Input: part model. Units: mm. Frame: model coordinates. Face numbers are marked on the shaded views. A direction names the side the tool comes from. Give positions to 0.01 mm unless a question says otherwise; leave off trailing zeros. Loops run counter-clockwise (first coordinate to the right, second up) from the corner with the lowest first, then second, coordinate; pieces in that order, holes last. Notation, with made-up numbers: (25, 50) -> (82, 50) arc R23 ccw to (82, 79) -> close; hole circle Ø8 at (6, 77.25). An arc over 180 degrees is marked (long way). One line per question, with ' | ' between items.
from build123d import *

# Parameters (mm, degrees)
F0_W     = 44
F0_H     = 44
F1_DEPTH = 25
F0_W_2   = 264
F0_H_2   = 264
F4_DEPTH = 50
F5_DEPTH = 44
F6_DEPTH = 22
F7_SIZE  = 21.99999


# Not quite as in the source:
# - a fillet or chamfer is up to 0.001 mm smaller than in the source, because OpenCascade refuses the exact size


with BuildPart() as f1:
    # F0 (on Top) → F1 (new body)
    with BuildSketch(Plane.XY):
        with Locations((-88, 88)):
            Rectangle(F0_W, F0_H)
    extrude(amount=F1_DEPTH)


with BuildPart() as f1b:
    # F0 (on Top) → F1, piece 2 (new body)
    with BuildSketch(Plane.XY):
        with Locations((0, 88)):
            Rectangle(F0_W, F0_H)
    extrude(amount=F1_DEPTH)


with BuildPart() as f1c:
    # F0 (on Top) → F1, piece 3 (new body)
    with BuildSketch(Plane.XY):
        Rectangle(F0_W, F0_H)
    extrude(amount=F1_DEPTH)


with BuildPart() as f1d:
    # F0 (on Top) → F1, piece 4 (new body)
    with BuildSketch(Plane.XY):
        with Locations((-88, 0)):
            Rectangle(F0_W, F0_H)
    extrude(amount=F1_DEPTH)


with BuildPart() as f2_1:
    # F2: instance of F1d
    add(f1d.part.mirror(Plane.YZ))


with BuildPart() as f2_2:
    # F2: instance of F1
    add(f1.part.mirror(Plane.YZ))


with BuildPart() as f3_1:
    # F3: instance of F1
    add(f1.part.mirror(Plane.XZ))


with BuildPart() as f3_2:
    # F3: instance of F1b
    add(f1b.part.mirror(Plane.XZ))


with BuildPart() as f3_3:
    # F3: instance of F2_2
    add(f2_2.part.mirror(Plane.XZ))


with BuildPart() as f1_1:
    add(f1.part)

    add(f1b.part)  # F4 merges F1b

    add(f1c.part)  # F4 merges F1c

    add(f1d.part)  # F4 merges F1d

    add(f2_1.part)  # F4 merges F2_1

    add(f2_2.part)  # F4 merges F2_2

    add(f3_1.part)  # F4 merges F3_1

    add(f3_2.part)  # F4 merges F3_2

    add(f3_3.part)  # F4 merges F3_3
    # F0 (on Top) → F4 (join)
    with BuildSketch(Plane.XY):
        Rectangle(F0_W_2, F0_H_2)
        with Locations((-88, 0)):
            Rectangle(F0_W, F0_H, mode=Mode.SUBTRACT)
        with Locations((-88, 88)):
            Rectangle(F0_W, F0_H, mode=Mode.SUBTRACT)
        Rectangle(F0_W, F0_H, mode=Mode.SUBTRACT)
        with Locations((0, 88)):
            Rectangle(F0_W, F0_H, mode=Mode.SUBTRACT)
        with Locations((-88, 0)):
            Rectangle(F0_W, F0_H)
        Rectangle(F0_W, F0_H)
        with Locations((-88, 88)):
            Rectangle(F0_W, F0_H)
        with Locations((0, 88)):
            Rectangle(F0_W, F0_H)
    extrude(amount=-F4_DEPTH)

    # F5 (add): faces of the model
    f5_faces = [f1_1.faces().sort_by_distance(p)[0] for p in [
        (-88, -66, 12.5),
        (-88, 22, 12.5),
        (0, 22, 12.5),
        (0, -66, 12.5),
        (88, -66, 12.5),
        (88, 22, 12.5),
    ]]
    extrude(f5_faces, amount=F5_DEPTH)

    # F6 (add, symmetric): faces of the model
    f6_faces = [f1_1.faces().sort_by_distance(p)[0] for p in [
        (-88, -110, 12.5),
        (0, -110, 12.5),
        (88, -110, 12.5),
        (-88, 110, 12.5),
        (0, 110, 12.5),
        (88, 110, 12.5),
    ]]
    extrude(f6_faces, amount=F6_DEPTH, both=True, dir=(0, -1, 0))

    # F7 (size 22 in the source; OpenCascade refuses exactly that, so slightly less here)
    f7_edges = [f1_1.edges().sort_by_distance(p)[0] for p in [
        (-110, 0, 25),
        (-66, 0, 25),
        (-22, 0, 25),
        (22, 0, 25),
        (110, 0, 25),
        (66, 0, 25),
    ]]
    chamfer(f7_edges, length=F7_SIZE)


solid = f1_1.part
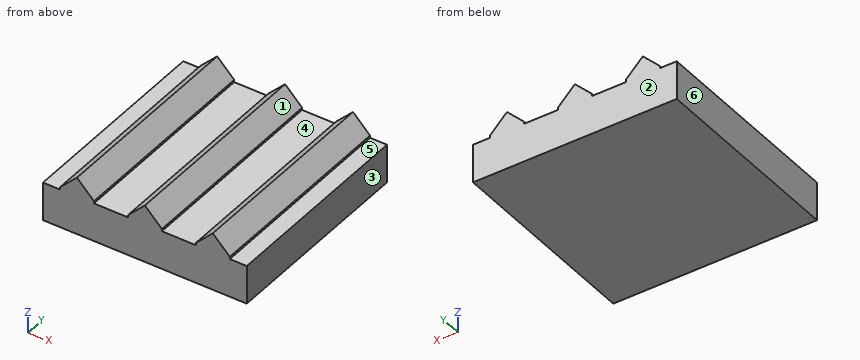
1. Ray query, line 1 along X through (y, z) = (-88, 1); line 2 along X through (y, z) = (37, 19); line 3 along Z through (x, y) = (39, 43). Return the intervals inside material, ascending. Write a range as from..to.
Determined:
line 1: x = -110..-66, -22..22, 66..110 | line 2: x = -94..-82, -6..6, 82..94 | line 3: z = -50..0
2. Section query C-C (x = 80). Output: boundary loops of the cut face in (y, z), then the cut area to 3 significant figures.
Determined:
outline: (-132, -50) -> (132, -50) -> (132, 17) -> (-132, 17) -> close | area: 17,700 mm2
3. Pull-direction query (X, two-part tool) for the marked faces 3, 4, 5 and 6; classes: pulls with the +X half, pulls with the -X half, needs draft (parallel to the pull), parting line crosses it, or undercut.
Determined:
face 3: pulls with the +X half | face 4: undercut | face 5: needs draft | face 6: pulls with the -X half
4. Pin query (flat end, axial travel): P1, Ø13, axis at x = -42.5, y = 10.5, coming from the +Z side; P2, Ø2.5, axis at y = 65.5, z = 2, coming from the +X side; P3, Ø1.5, axis at y = -30, z = 1, coming from the -X side. Return the tip coordinate at first contact, or that it passes through.
Determined:
P1: stops at z = 0 | P2: stops at x = 110 | P3: stops at x = -110
5. Section query B-B (x = 51.5). Output: boundary loops of the cut face in (y, z), then the cut area to 3 significant figures.
Determined:
outline: (-132, -50) -> (132, -50) -> (132, 0) -> (-132, 0) -> close | area: 13,200 mm2
6. Reachability of the marked faces 1 and 2 from +Z, -Z, +X, -X, +Y, -Y: full face, straight path, thin tool, end or side. Return the list, or none.
Determined:
face 1: +Z, +Y, -Y | face 2: +Z, -Z, +X, -X, +Y
